Verification items for the finished model (mm, model axes). Face numbers are marked on the shaded views. A direction names the side the tool comes from. Coordinates: 2 decimals unless noted, no trailing zeros. Write each loop counter-clockwise with the first axis right and the second up, starting at its lowest first coordinate (ties: lowest second). Pieces come first, ordered by that corner, then holes. Notation, with made-up numbers: (-9, 85.25) -> (-1, 85.25) arc R16 cw to (-1, 105.25) -> close; hole circle Ø6 at (-30.75, 66.5). An arc over 180 degrees is marked (long way). Use CSV: the item, a comma, the result in double quotes.
```python
from build123d import *

# Parameters (mm, degrees)
CROQUIS1_R                   = 1.5
SALIENTE_EXTRUIR1_DEPTH      = 3.5
SALIENTE_EXTRUIR2_DEPTH      = 2.5
SALIENTE_EXTRUIR2_DEPTH_BACK = 3.5
CROQUIS3_R                   = 1.625
CORTAR_EXTRUIR1_DEPTH        = 2.5
CORTAR_EXTRUIR2_DEPTH        = 2.5
CROQUIS6_W                   = 4
CROQUIS6_H                   = 8.575
SALIENTE_EXTRUIR4_DEPTH      = 2.5


with BuildPart() as part:
    # Croquis1 → Saliente-Extruir1 (new body)
    with BuildSketch(Plane.XY):
        Polygon((168.732371, -66.648646), (161.232371, -66.648646), (161.232371, -80.148646), (167.387371, -80.148646), (168.732371, -81.493646), (168.732371, -80.148646), align=None)
        with Locations((165.232371, -75.223646)):
            Circle(CROQUIS1_R, mode=Mode.SUBTRACT)
    extrude(amount=SALIENTE_EXTRUIR1_DEPTH)

    # Croquis3 → Saliente-Extruir2 (add, two sides: drawn at the far end of the back side and taken through both)
    with BuildSketch(Plane.XY.offset(3.5).offset(-SALIENTE_EXTRUIR2_DEPTH_BACK)):
        Polygon((168.732371, -81.493646), (181.732371, -81.493646), (181.732371, -74.071146), (173.47767153, -66.648646), (173.47767153, -75.223646), (169.47767153, -75.223646), (169.47767153, -66.648646), (168.732371, -66.648646), align=None)
        with Locations((177.73707047, -75.223646)):
            Circle(CROQUIS3_R, mode=Mode.SUBTRACT)
    extrude(amount=SALIENTE_EXTRUIR2_DEPTH + SALIENTE_EXTRUIR2_DEPTH_BACK)

    # Croquis4 → Cortar-Extruir1 (cut)
    with BuildSketch(Plane.XY.offset(6)):
        Polygon((177.73707047, -78.393646), (180.482371, -76.808646), (180.482371, -73.638646), (177.73707047, -72.053646), (174.99176994, -73.638646), (174.99176994, -76.808646), align=None)
    extrude(amount=-CORTAR_EXTRUIR1_DEPTH, mode=Mode.SUBTRACT)

    # Croquis5 → Cortar-Extruir2 (cut)
    with BuildSketch(Plane.XY.offset(3.5)):
        Polygon((165.232371, -78.393646), (167.97767153, -76.808646), (167.97767153, -73.638646), (165.232371, -72.053646), (162.48707047, -73.638646), (162.48707047, -76.808646), align=None)
    extrude(amount=-CORTAR_EXTRUIR2_DEPTH, mode=Mode.SUBTRACT)

    # Croquis6 → Saliente-Extruir4 (add)
    with BuildSketch(Plane.XY.offset(6)):
        with Locations((171.47767153, -70.936146)):
            Rectangle(CROQUIS6_W, CROQUIS6_H)
    extrude(amount=-SALIENTE_EXTRUIR4_DEPTH)


solid = part.part
```
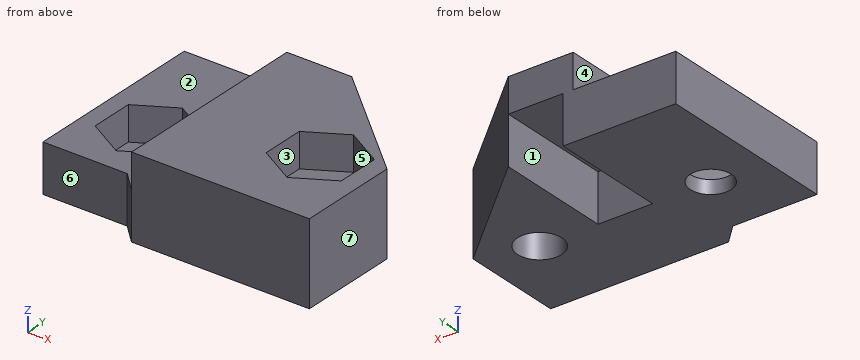
1) Set-up check for the marked faces 1, 2 and 3: record each of +Z, -Z, +X, -X, +Y, -Y from which the full face is reachable in a straight line by a thin tool's end or side.
Return value:
face 1,"-Z, +Y"
face 2,"+Z, -X, +Y, -Y"
face 3,"+Z"
2) Cross-section at B-B (z = 4.15). Record the boundary of the cut face in (x, y), plus the area to 3 significant figures.
Return value:
outline,"(168.73, -81.49) -> (181.73, -81.49) -> (181.73, -74.07) -> (173.48, -66.65) -> (168.73, -66.65) -> close; hole (174.99, -76.81) -> (177.74, -78.39) -> (180.48, -76.81) -> (180.48, -73.64) -> (177.74, -72.05) -> (174.99, -73.64) -> close"
area,"136 mm2"
3) Cross-section at A-A (z = 0.4). Record the boundary of the cut face in (x, y) (3 decimals), plus the area to 3 significant figures.
Return value:
outline,"(161.232, -80.149) -> (167.387, -80.149) -> (168.732, -81.494) -> (181.732, -81.494) -> (181.732, -74.071) -> (173.478, -66.649) -> (173.478, -75.224) -> (169.478, -75.224) -> (169.478, -66.649) -> (161.232, -66.649) -> close; hole circle Ø3 at (165.232, -75.224); hole circle Ø3.25 at (177.737, -75.224)"
area,"215 mm2"
4) Scan lines: L1, parallel to X at y = -75.5, z = 5.7; L2, parallel to Z at x = 166, y = -73.5; L3, parallel to Y at x = 178.5, z = 0.65. Record each from-to range of solid material in increasing order.
Return value:
L1,"168.73 to 174.99, 180.48 to 181.73"
L2,"0 to 1"
L3,"-81.49 to -76.66, -73.79 to -71.16"
5) Cross-section at D-D (y = -70). Record the boundary of the cut face in (x, z), plus the area to 3 significant figures.
Return value:
outline,"(161.23, 0) -> (169.48, 0) -> (169.48, 3.5) -> (173.48, 3.5) -> (173.48, 0) -> (177.2, 0) -> (177.2, 6) -> (168.73, 6) -> (168.73, 3.5) -> (161.23, 3.5) -> close"
area,"63.1 mm2"
6) Mould release check, pull along X, two halves, no side actions. Record for the marked faces 4, 5, 6 and 7: released by +X, released by -X, zero draft, split by the parting line, or undercut.
Return value:
face 4,"released by -X"
face 5,"undercut"
face 6,"zero draft"
face 7,"released by +X"
7) Cross-section at C-C (x = 178). Record the boundary of the cut face in (y, z).
Return value:
outline,"(-81.49, 0) -> (-76.83, 0) -> (-76.83, 3.5) -> (-78.24, 3.5) -> (-78.24, 6) -> (-81.49, 6) -> close; (-73.62, 0) -> (-70.72, 0) -> (-70.72, 6) -> (-72.21, 6) -> (-72.21, 3.5) -> (-73.62, 3.5) -> close"
8) Gauge pin test, flat ends, axial feed: pin 1 (1.2 mm diameter, centred on x = 171, y = -72, fed in from -Z); pin 2 (5 mm diameter, centred on x = 177.74, y = -75.22, fed in from +Z); pin 3 (1.6 mm diameter, centred on x = 165.5, y = -76, fed in from +Z). Record the tip position at first contact, or that the pin passes through.
Return value:
pin 1,"z = 3.5"
pin 2,"z = 3.5"
pin 3,"z = 1"
